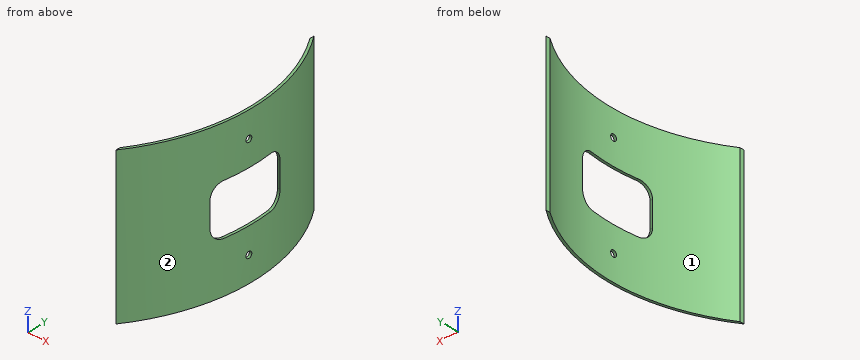
```python
from build123d import *

# Parameters (mm, degrees)
BOSS_EXTRU_1_DEPTH                = 120
DIAM_TRE_DU_PER_AGE_5_0_5_1_D     = 5
DIAM_TRE_DU_PER_AGE_5_0_5_1_DEPTH = 60
DIAM_TRE_DU_PER_AGE_5_0_5_1_TIP   = 1.502151548
ENL_V_MAT_EXTRU_2_DEPTH           = 208.889393843


with BuildPart() as part:
    # Esquisse1 → Boss.-Extru.1 (new body)
    with BuildSketch(Plane.XY):
        with BuildLine():
            Line((120, 84.905830189), (120, 81.39410298))
            ThreePointArc((120, 81.39410298), (145, 0), (120, -81.39410298))
            Line((120, -81.39410298), (120, -84.905830189))
            ThreePointArc((120, -84.905830189), (147, 0), (120, 84.905830189))
        make_face()
    extrude(amount=BOSS_EXTRU_1_DEPTH)

    # Diamètre du perçage Ø5.0 (5)1
    with Locations(Plane(origin=(147, 0, 20), x_dir=(0, 1, 0), z_dir=(1, 0, 0))):
        with Locations((0, 0), (0, 80)):
            Hole(DIAM_TRE_DU_PER_AGE_5_0_5_1_D / 2, depth=DIAM_TRE_DU_PER_AGE_5_0_5_1_DEPTH)
            with Locations((0, 0, -(DIAM_TRE_DU_PER_AGE_5_0_5_1_DEPTH + DIAM_TRE_DU_PER_AGE_5_0_5_1_TIP / 2))):  # 118° drill point
                Cone(0, DIAM_TRE_DU_PER_AGE_5_0_5_1_D / 2, DIAM_TRE_DU_PER_AGE_5_0_5_1_TIP, mode=Mode.SUBTRACT)

    # Esquisse3 → Enlèv. mat.-Extru.2 (cut, through all)
    with BuildSketch(Plane(origin=(0, 0, 0), x_dir=(0, 0, -1), z_dir=(1, 0, 0))):
        with BuildLine():
            Line((-70, 30), (-50, 30))
            ThreePointArc((-50, 30), (-42.928932188, 27.071067812), (-40, 20))
            Line((-40, 20), (-40, -20))
            ThreePointArc((-40, -20), (-42.928932188, -27.071067812), (-50, -30))
            Line((-50, -30), (-70, -30))
            ThreePointArc((-70, -30), (-77.071067812, -27.071067812), (-80, -20))
            Line((-80, -20), (-80, 20))
            ThreePointArc((-80, 20), (-77.071067812, 27.071067812), (-70, 30))
        make_face()
    extrude(amount=ENL_V_MAT_EXTRU_2_DEPTH, mode=Mode.SUBTRACT)


solid = part.part
```
Work out the finished part from the listing and answer in its coordinate system (mm). Face numbers are marked on the shaded views. Coordinates: 2 decimals unless noted, no trailing zeros. Loops run counter-clockwise (first coordinate to the right, second up) from the corner with the lowest first, then second, coordinate; pieces in that order, holes last. Notation, with made-up numbers: (-24, 10.25) - (0, 10.25) arc R33 ccw to (0, 45.25) - close; hole circle Ø1 at (57.5, 48.25). An arc over 180 degrees is marked (long way). Use a Markdown table: item, result.
Item 1: The mould has two halves that part along Y. Classify the marked faces 1 and 2: +Y half, -Y half, draft (parallel to the pull), parting line (faces both ways), or undercut.
Evaluation:
| item | result |
|---|---|
| face 1 | undercut |
| face 2 | parting line |
Item 2: Find section C-C, the plane z = 76. Determine the outline of the cut face in (x, y).
Evaluation:
| item | result |
|---|---|
| outline | (120, -84.91) arc R147 ccw to (144.31, -28) - (142.27, -28) arc R145 cw to (120, -81.39) - close; (120, 81.39) arc R145 cw to (142.27, 28) - (144.31, 28) arc R147 ccw to (120, 84.91) - close |
Item 3: Consider probe 1 along Z at (x, y) = (146.3, 0); probe 2 along Y at (x, z) = (133.5, 83); probe 3 along Y at (x, z) = (126.75, 110.5). Determine where each line is inside the solid, lowest interval first. Write a range as from..to.
Evaluation:
| item | result |
|---|---|
| probe 1 | z = 0..17.5, 22.5..40, 80..97.5, 102.5..120 |
| probe 2 | y = -61.54..-56.59, 56.59..61.54 |
| probe 3 | y = -74.45..-70.42, 70.42..74.45 |
Item 4: Find section A-A, the plane y = 0. Determine the outline of the cut face in (x, z), and give its area (3 significant figures).
Evaluation:
| item | result |
|---|---|
| outline | (145, 0) - (147, 0) - (147, 17.5) - (145, 17.5) - close; (145, 22.5) - (147, 22.5) - (147, 40) - (145, 40) - close; (145, 80) - (147, 80) - (147, 97.5) - (145, 97.5) - close; (145, 102.5) - (147, 102.5) - (147, 120) - (145, 120) - close |
| area | 140 mm2 |
Item 5: Find section B-B, the plane x = 126.5. Determine the outline of the cut face in (y, z).
Evaluation:
| item | result |
|---|---|
| outline | (-74.88, 0) - (-70.87, 0) - (-70.87, 120) - (-74.88, 120) - close; (70.87, 0) - (74.88, 0) - (74.88, 120) - (70.87, 120) - close |
Item 6: Find section D-D, the plane z = 11. Determine the outline of the cut face in (x, y).
Evaluation:
| item | result |
|---|---|
| outline | (120, -84.91) arc R147 ccw to (120, 84.91) - (120, 81.39) arc R145 cw to (120, -81.39) - close |
Item 7: Given pin 1 Ø2 at (x, z) = (133, 23) entering from +Y; pin 2 Ø1.5 at (x, z) = (137, 81.5) entering from -Y; pin 3 Ø4.5 at (y, z) = (0, 20) entering from +X; pin 4 Ø10 at (x, z) = (133.5, 67.5) entering from +Y, each flat-ended and moving along its own axis, determine where each tip first touches the part or whether it passes through.
Evaluation:
| item | result |
|---|---|
| pin 1 | stops at y = 64.69 |
| pin 2 | stops at y = -55.18 |
| pin 3 | passes through |
| pin 4 | stops at y = 71.39 |
